Part model, mm, in its own coordinate system. Face numbers are marked on the shaded views. A direction names the side the tool comes from. Coordinates: 2 decimals unless noted, no trailing zeros. Loops run counter-clockwise (first coordinate to the right, second up) from the corner with the lowest first, then second, coordinate; pieces in that order, holes last. Notation, with made-up numbers: M -23,19 L -15,19 A33 cw -15,56 Z; hole C 30.5,28.25 d2. An arc over 180 degrees is marked long. Answer as a JSON object with one key per item and string values. Group by question number.
1. Saw through at D-D on y = -17. Write the cut outline in (x, z), then the cut area to 3 significant figures.
2. Saw through at C-C on x = -4. Write the cut outline in (y, z).
3. Saw through at A-A on x = 5. Write the cut outline in (y, z).
4. Mould opens along Y. For the marked faces 1, 2 and 3 say: released by +Y, released by -Y, zero draft, split by the parting line, or undercut.
5. Drill centre lines: L1, parallel to Z at x = 1, y = 9; L2, parallel to Y at x = -1, z = 26; L3, parallel to Y at x = -17.5, z = 43.5. Where is each one in solid material? Low to high.
6. 3-axis set-ups, long thin cutter, end or side, ignore diameter. For the marked faces 4, 5, 6, 7 and 8: which of +Z, -Z, +X, -X, +Y, -Y reach the whole face in a straight line?
7. Saw through at B-B on y = -36. Write the cut outline in (x, z), then the cut area to 3 significant figures.
8. Drop flat-ended pins along their axis: pin 1 Ø16 at (x, y) = (-4, -39) entering from +Z; pin 2 Ø2 at (x, z) = (1.5, 29.5) entering from -Y; pin 3 Ø12 at (y, z) = (-10, 41) entering from +X; pin 4 Ø17.5 at (y, z) = (-41.5, 21.5) entering from -X. Give the stop position or say it passes through.
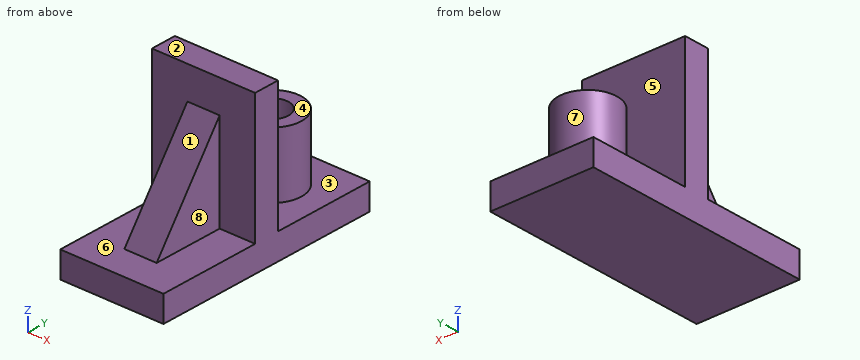
from build123d import *

# Parameters (mm, degrees)
SKETCH2_W           = 32
SKETCH2_H           = 72
BOSS_EXTRUDE1_DEPTH = 8
SKETCH3_R           = 9
SKETCH3_R_2         = 5
SKETCH3_W           = 32
SKETCH3_H           = 8
BOSS_EXTRUDE2_DEPTH = 20
SKETCH4_W           = 32
SKETCH4_H           = 8
BOSS_EXTRUDE3_DEPTH = 20
RIB1_REACH          = 80.09
SKETCH5_WALL_W      = 195.381659614
SKETCH5_WALL_H      = 10


with BuildPart() as part:
    # Sketch2 → Boss-Extrude1 (new body)
    with BuildSketch(Plane.XY):
        with Locations((-4.753138075, -23.481171548)):
            Rectangle(SKETCH2_W, SKETCH2_H)
    extrude(amount=BOSS_EXTRUDE1_DEPTH)

    # Sketch3 → Boss-Extrude2 (add)
    # profile 1 of 2: a face of its own
    with BuildSketch(Plane.XY.offset(8)):
        with Locations((-4.753138075, -3.481171548)):
            Circle(SKETCH3_R)
        with Locations((-4.753138075, -3.481171548)):
            Circle(SKETCH3_R_2, mode=Mode.SUBTRACT)
    # profile 2 of 2: a face of its own
    with BuildSketch(Plane.XY.offset(8)):
        with Locations((-4.753138075, -23.481171548)):
            Rectangle(SKETCH3_W, SKETCH3_H)
    extrude(amount=BOSS_EXTRUDE2_DEPTH)

    # Sketch4 → Boss-Extrude3 (add)
    with BuildSketch(Plane.XY.offset(28)):
        with Locations((-4.753138075, -23.481171548)):
            Rectangle(SKETCH4_W, SKETCH4_H)
    extrude(amount=BOSS_EXTRUDE3_DEPTH)

    # Sketch5 wall → Rib1 (add, up to next)
    with BuildSketch(Plane(origin=(-4.753138075, -38.481171548, 23), x_dir=(0, -0.591363663628, -0.806404995856), z_dir=(0, -0.806404995856, 0.591363663628)), mode=Mode.PRIVATE) as rib1_sk1:
        Rectangle(SKETCH5_WALL_W, SKETCH5_WALL_H)
    rib1_tool1 = extrude(rib1_sk1.sketch, amount=-RIB1_REACH, mode=Mode.PRIVATE) - part.part
    add(rib1_tool1.solids().sort_by_distance((-4.753138075, -38.481171548, 23))[0])


solid = part.part
Outcome:
{
 "1": {"outline": "M -20.75,0 L 11.25,0 L 11.25,8 L -20.75,8 Z", "area": "256 mm²"},
 "2": {"outline": "M -59.48,0 L 12.52,0 L 12.52,8 L 5.49,8 L 5.49,28 L 1.46,28 L 1.46,8 L -8.42,8 L -8.42,28 L -12.45,28 L -12.45,8 L -19.48,8 L -19.48,48 L -27.48,48 L -27.48,38 L -49.48,8 L -59.48,8 Z"},
 "3": {"outline": "M -59.48,0 L 12.52,0 L 12.52,8 L -19.48,8 L -19.48,48 L -27.48,48 L -27.48,8 L -59.48,8 Z"},
 "4": {"face 1": "released by -Y", "face 2": "zero draft", "face 3": "undercut"},
 "5": {"L1": "z = 0 to 8", "L2": "y = -36.28 to -19.48, -11.66 to -6.78, -0.18 to 4.7", "L3": "y = -27.48 to -19.48"},
 "6": {"face 4": "+Z, +X, -X, +Y", "face 5": "+Z, +X, -X", "face 6": "+Z, -Y", "face 7": "+Z", "face 8": "+Z, +X, -Y"},
 "7": {"outline": "M -20.75,0 L 11.25,0 L 11.25,8 L 0.25,8 L 0.25,26.38 L -9.75,26.38 L -9.75,8 L -20.75,8 Z", "area": "440 mm²"},
 "8": {"pin 1": "stops at z = 33.2", "pin 2": "stops at y = -27.48", "pin 3": "passes through", "pin 4": "stops at x = -9.75"}
}
